Source: CAD feature listing. Evaluate the final solid. Frame: model axes, mm. A direction names the side the tool comes from. Round coordinates to 2 decimals unless told otherwise and drop trailing zeros. Loops run counter-clockwise (first coordinate to the right, second up) from the corner with the lowest first, then second, coordinate; pieces in that order, holes last. Notation, with made-up numbers: M 5.25,-38.5 L 33.25,-38.5 A26 ccw 33.25,-6.5 Z; hole C 22.5,-12.75 d9. An arc over 180 degrees is marked long. One line per item, written item: value.
from build123d import *

# Parameters (mm, degrees)
F0_W      = 762
F0_H      = 1016
F1_DEPTH  = 19.05
F2_W      = 101.6
F2_H      = 1016
F3_DEPTH  = 76.2
F4_W      = 152.4
F4_H      = 1016
F5_DEPTH  = 19.05
F6_W      = 812.8
F6_H      = 1016
F7_DEPTH  = 19.05
F8_W      = 101.6
F8_H      = 1016
F9_DEPTH  = 19.05
F10_W     = 19.05
F10_H     = 431.8
F10_W_2   = 387.35
F10_H_2   = 19.05
F10_W_3   = 368.3
F11_DEPTH = 107.95


with BuildPart() as f1:
    # F0 (on Top) → F1 (new body)
    with BuildSketch(Plane.XY):
        with Locations((381, 508)):
            Rectangle(F0_W, F0_H)
    extrude(amount=F1_DEPTH)

    # F2 (on face) → F3 (join)
    with BuildSketch(Plane.XY.offset(19.05)):
        with Locations((50.8, 508)):
            Rectangle(F2_W, F2_H)
        with Locations((711.2, 508)):
            Rectangle(F2_W, F2_H)
    extrude(amount=F3_DEPTH)

    # F4 (on face) → F5 (join)
    with BuildSketch(Plane.XY.offset(95.25)):
        with Locations((736.6, 508)):
            Rectangle(F4_W, F4_H)
    extrude(amount=F5_DEPTH)

    # F6 (on face) → F7 (join)
    with BuildSketch(Plane(origin=(0, 0, 0), x_dir=(1, 0, 0), z_dir=(0, 0, -1))):
        with Locations((406.4, -508)):
            Rectangle(F6_W, F6_H)
    extrude(amount=F7_DEPTH)

    # F8 (on face) → F9 (join)
    with BuildSketch(Plane.XY.offset(95.25)):
        with Locations((50.8, 508)):
            Rectangle(F8_W, F8_H)
    extrude(amount=F9_DEPTH)

    # F10 (on face) → F11 (join)
    with BuildSketch(Plane(origin=(0, 0, -19.05), x_dir=(1, 0, 0), z_dir=(0, 0, -1))):
        with Locations((9.525, -215.9)):
            Rectangle(F10_W, F10_H)
        Polygon((19.05, -431.8), (0, -431.8), (0, -450.85), (19.05, -450.85), (406.4, -450.85), (425.45, -450.85), (793.75, -450.85), (812.8, -450.85), (812.8, -431.8), (793.75, -431.8), align=None)
        with Locations((803.275, -215.9)):
            Rectangle(F10_W, F10_H)
        with Locations((212.725, -460.375)):
            Rectangle(F10_W_2, F10_H_2)
        Polygon((425.45, -450.85), (406.4, -450.85), (406.4, -469.9), (406.4, -714.375), (406.4, -733.425), (406.4, -996.95), (425.45, -996.95), (425.45, -733.425), (425.45, -714.375), (425.45, -469.9), align=None)
        with Locations((609.6, -460.375)):
            Rectangle(F10_W_3, F10_H_2)
        with Locations((212.725, -723.9)):
            Rectangle(F10_W_2, F10_H_2)
        with Locations((609.6, -723.9)):
            Rectangle(F10_W_3, F10_H_2)
        Polygon((425.45, -996.95), (406.4, -996.95), (19.05, -996.95), (19.05, -1016), (793.75, -1016), (793.75, -996.95), align=None)
    extrude(amount=F11_DEPTH)


solid = f1.part
1. Section query C-C (y = 345). Return the cut outline in (x, z), and give its area (3 significant figures).
Report:
outline: M 0,-127 L 19.05,-127 L 19.05,-19.05 L 793.75,-19.05 L 793.75,-127 L 812.8,-127 L 812.8,0 L 762,0 L 762,95.25 L 812.8,95.25 L 812.8,114.3 L 660.4,114.3 L 660.4,19.05 L 101.6,19.05 L 101.6,114.3 L 0,114.3 Z
area: 54,400 mm2
2. Pull-direction query (Y, two-part tool) for faces 1 (the face through (812.8, 289, -63)), 2 (the face through (406.4, 863, -72)), 3 (the face through (405, 0, 3)); classes: released by +Y, released by -Y, zero draft, split by the parting line, or undercut.
Report:
face 1: zero draft
face 2: undercut
face 3: released by -Y
3. Section query B-B (z = -101). Return the cut outline in (x, y) (3 decimals), and give its area (3 significant figures).
Report:
outline: M 0,0 L 19.05,0 L 19.05,431.8 L 793.75,431.8 L 793.75,0 L 812.8,0 L 812.8,450.85 L 793.75,450.85 L 793.75,469.9 L 425.45,469.9 L 425.45,714.375 L 793.75,714.375 L 793.75,733.425 L 425.45,733.425 L 425.45,996.95 L 793.75,996.95 L 793.75,1016 L 19.05,1016 L 19.05,996.95 L 406.4,996.95 L 406.4,733.425 L 19.05,733.425 L 19.05,714.375 L 406.4,714.375 L 406.4,469.9 L 19.05,469.9 L 19.05,450.85 L 0,450.85 Z
area: 85,900 mm2
4. Pin query (flat end, axial travel): pin 1 (1.5 mm diameter, centred on x = 341, y = 401, fed in from -Z); pin 2 (12 mm diameter, centred on x = 519, y = 649.5, fed in from +Z); pin 3 (15 mm diameter, centred on x = 806, z = -71.5, fed in from +Y). Return the tip coordinate at first contact, or that it passes through.
Report:
pin 1: stops at z = -19.05
pin 2: stops at z = 19.05
pin 3: stops at y = 450.85
5. Reachability of faces 4 (the face through (607, 733.425, -72)), 5 (the face through (401, 213, -19.05)), 6 (the face through (660.4, 501, 66)) from +Z, -Z, +X, -X, +Y, -Y: full face, straight path, thin tool, end or side. Return the list, or none.
Report:
face 4: -Z, +X
face 5: -Z, -Y
face 6: +Z, +Y, -Y
6. Section query D-D (z = 72). Return the cut outline in (x, y).
Report:
outline: M 0,0 L 101.6,0 L 101.6,1016 L 0,1016 Z; M 660.4,0 L 762,0 L 762,1016 L 660.4,1016 Z
7. Section query A-A (x = 442). Return the cut outline in (y, z) (3 decimals), and give its area (3 significant figures).
Report:
outline: M 0,-19.05 L 431.8,-19.05 L 431.8,-127 L 469.9,-127 L 469.9,-19.05 L 714.375,-19.05 L 714.375,-127 L 733.425,-127 L 733.425,-19.05 L 996.95,-19.05 L 996.95,-127 L 1016,-127 L 1016,19.05 L 0,19.05 Z
area: 46,900 mm2
8. Ray query, line 1 (Y direction, x = 756.5, z = -49.5) (3 decimals); line 2 (Z direction, x = 763, y = 451); line 3 (X direction, y = 909.5, z = 70). Return the intervals inside material, ascending. Write a range as [from, to].
Report:
line 1: y = [431.8, 469.9], [714.375, 733.425], [996.95, 1016]
line 2: z = [-127, 0], [95.25, 114.3]
line 3: x = [0, 101.6], [660.4, 762]
